Read the model definition and answer for the solid it produces. Units are mm, in the model's axes. A direction names the side the tool comes from. Give positions to 0.01 mm unless a question says otherwise; leave off trailing zeros. Write each loop counter-clockwise with the first axis right and the second up, starting at its lowest first coordinate (ties: lowest second). Pieces come first, ordered by that corner, then holes. Notation, with made-up numbers: (56.25, 28) - (85.25, 28) arc R21 ccw to (85.25, 52) - close; hole circle Ø8 at (63.25, 61). An arc over 180 degrees is marked (long way). Answer as CSV lines item,"result".
```python
from build123d import *


with BuildPart() as part:
    # 草图1 → 旋转2 (revolve)
    with BuildSketch(Plane.XY, mode=Mode.PRIVATE) as revolve_2_sk:
        Polygon((14.5, 27.042854175), (15, 27.042854175), (15.5, 26.542854175), (15.5, 2.642854175), (15, 2.642854175), (15, 1.642854175), (18.55, 1.642854175), (19.05, 1.142854175), (19.05, -5.357145825), (18.55, -5.857145825), (18, -5.857145825), (17.5, -5.357145825), (17.5, -1.357145825), (17.6, -1.357145825), (17.6, -0.357145825), (14, -0.357145825), (14, 26.542854175), align=None)
    revolve(revolve_2_sk.sketch.rotate(Axis((0, 44.598597745, 0), (0, -1, 0)), 90), axis=Axis((0, 44.598597745, 0), (0, -1, 0)))  # turned: the seam where the file's is


solid = part.part
```
(1) For faces 1 (the flat face through (14, 1.643, -7)), 2 (the cylindrical face through (-15.368, 14.426, -2.018)), 3 (the cylindrical face through (12.4, 13.3, 6.5)), determine the directions among +Z, -Z, +X, -X, +Y, -Y from which every point of the face is accessible in a straight line to the end or side of a thin tool.
Worked out:
face 1,"none"
face 2,"+Y"
face 3,"+Y, -Y"
(2) A cutting plane is placed at C-C (y = 15.5). Write down the section's boundary in (x, z), and give its area (3 significant figures).
Worked out:
outline,"circle Ø31 at (0, 0); hole circle Ø28 at (0, 0)"
area,"139 mm^2"
(3) A cutting plane is placed at D-D (y = -3). Write down the section's boundary in (x, z).
Worked out:
outline,"circle Ø38.1 at (0, 0); hole circle Ø35 at (0, 0)"
(4) The mould has two halves that part along Y. Classify faces 4 (the cylindrical face through (17.084, -3.329, -3.794)), 5 (the cylindrical face through (-17.45, -0.85, -2.29)), 6 (the cylindrical face through (-12.65, 2.14, 8.06)), 7 (the flat face through (-18, -5.857, -3)): +Y half, -Y half, draft (parallel to the pull), parting line (faces both ways), or undercut.
Worked out:
face 4,"draft"
face 5,"undercut"
face 6,"undercut"
face 7,"-Y half"
(5) Each of these flat-tipped pins is pushed along its axis until it touches: P1, Ø11, axis at x = -6, z = 3, coming from the +Y side; P2, Ø1, axis at y = 11.5, z = -5.5, coming from the +X side; P3, Ø8, axis at y = 5.5, z = -5.5, coming from the +X side; P4, Ø3, axis at y = 23, z = -6, coming from the -X side. Where does it stop, or does it pass through?
Worked out:
P1,"passes through"
P2,"stops at x = 14.67"
P3,"stops at x = 18.01"
P4,"stops at x = -14.83"
(6) Find the intervals of material crossed by L1, parallel to X at y = -1, z = 0; L2, parallel to X at y = -2.8, z = 0; L3, parallel to Z at x = -3.5, y = -4, in increasing order.
Worked out:
L1,"x = -19.05 to -17.6, 17.6 to 19.05"
L2,"x = -19.05 to -17.5, 17.5 to 19.05"
L3,"z = -18.73 to -17.15, 17.15 to 18.73"
